```python
from build123d import *

# Parameters (mm, degrees)
BOSS_EXTRUDE1_DEPTH = 22
SKETCH4_R           = 1.25
CUT_EXTRUDE1_DEPTH  = 3
BOSS_EXTRUDE2_DEPTH = 27
BOSS_EXTRUDE3_START = 27
BOSS_EXTRUDE3_DEPTH = 11.1
BOSS_EXTRUDE5_DEPTH = 23.5
SKETCH8_R           = 1.25
CUT_EXTRUDE2_DEPTH  = 3
SKETCH9_W           = 14
SKETCH9_H           = 10.1
CUT_EXTRUDE3_DEPTH  = 3


with BuildPart() as part:
    # Sketch3 → Boss-Extrude1 (new body)
    with BuildSketch(Plane.XY):
        with BuildLine():
            Line((-15, 3), (-4.369210455, 3))
            ThreePointArc((-4.369210455, 3), (0, 5.3), (4.369210455, 3))
            Line((4.369210455, 3), (15, 3))
            Line((15, 3), (15, 6))
            Line((15, 6), (5.734980384, 6))
            ThreePointArc((5.734980384, 6), (0, 8.3), (-5.734980384, 6))
            Line((-5.734980384, 6), (-15, 6))
            Line((-15, 6), (-15, 3))
        make_face()
    extrude(amount=BOSS_EXTRUDE1_DEPTH)

    # Sketch4 → Cut-Extrude1 (cut)
    with BuildSketch(Plane(origin=(0, 6, 0), x_dir=(1, 0, 0), z_dir=(0, 1, 0))):
        with Locations(Location((11.75, -18.75, 0), (0, 0, 180))):
            Circle(SKETCH4_R)
        with Locations(Location((11.75, -3.25, 0), (0, 0, 180))):
            Circle(SKETCH4_R)
        with Locations(Location((-11.75, -3.25, 0), (0, 0, 180))):
            Circle(SKETCH4_R)
        with Locations(Location((-11.75, -18.75, 0), (0, 0, 180))):
            Circle(SKETCH4_R)
    extrude(amount=-CUT_EXTRUDE1_DEPTH, mode=Mode.SUBTRACT)

    # Sketch5 → Boss-Extrude2 (add)
    with BuildSketch(Plane.XY.offset(22)):
        with BuildLine():
            Line((6, 4), (6, 3))
            Line((6, 3), (15, 3))
            Line((15, 3), (15, 6))
            Line((15, 6), (5.734980384, 6))
            ThreePointArc((5.734980384, 6), (0, 8.3), (-5.734980384, 6))
            Line((-5.734980384, 6), (-15, 6))
            Line((-15, 6), (-15, 3))
            Line((-15, 3), (-6, 3))
            Line((-6, 3), (-6, 4))
            ThreePointArc((-6, 4), (-5.707106781, 4.707106781), (-5, 5))
            Line((-5, 5), (-1.757839583, 5))
            ThreePointArc((-1.757839583, 5), (0, 5.3), (1.757839583, 5))
            Line((1.757839583, 5), (5, 5))
            ThreePointArc((5, 5), (5.707106781, 4.707106781), (6, 4))
        make_face()
        with BuildLine():
            ThreePointArc((-4.369210455, 3), (-3.222605397, 4.207708932), (-1.757839583, 5))
            Line((-1.757839583, 5), (-5, 5))
            ThreePointArc((-5, 5), (-5.707106781, 4.707106781), (-6, 4))
            Line((-6, 4), (-6, 3))
            Line((-6, 3), (-4.369210455, 3))
        make_face()
        with BuildLine():
            Line((4.369210455, 3), (6, 3))
            Line((6, 3), (6, 4))
            ThreePointArc((6, 4), (5.707106781, 4.707106781), (5, 5))
            Line((5, 5), (1.757839583, 5))
            ThreePointArc((1.757839583, 5), (3.222605397, 4.207708932), (4.369210455, 3))
        make_face()
    extrude(amount=BOSS_EXTRUDE2_DEPTH)

    # Sketch5<3> → Boss-Extrude3 (add)
    with BuildSketch(Plane.XY.offset(22).offset(BOSS_EXTRUDE3_START)):
        with BuildLine():
            Line((6, 4), (6, 3))
            Line((6, 3), (15, 3))
            Line((15, 3), (15, 6))
            Line((15, 6), (5.734980384, 6))
            ThreePointArc((5.734980384, 6), (0, 8.3), (-5.734980384, 6))
            Line((-5.734980384, 6), (-15, 6))
            Line((-15, 6), (-15, 3))
            Line((-15, 3), (-6, 3))
            Line((-6, 3), (-6, 4))
            ThreePointArc((-6, 4), (-5.707106781, 4.707106781), (-5, 5))
            Line((-5, 5), (-1.757839583, 5))
            ThreePointArc((-1.757839583, 5), (0, 5.3), (1.757839583, 5))
            Line((1.757839583, 5), (5, 5))
            ThreePointArc((5, 5), (5.707106781, 4.707106781), (6, 4))
        make_face()
    extrude(amount=BOSS_EXTRUDE3_DEPTH)

    # Sketch7 → Boss-Extrude5 (add)
    with BuildSketch(Plane.XY.offset(60.1)):
        with BuildLine():
            Line((-15, 6), (-15, 3))
            Line((-15, 3), (-6, 3))
            Line((-6, 3), (-6, 4))
            ThreePointArc((-6, 4), (-5.707106781, 4.707106781), (-5, 5))
            Line((-5, 5), (-1.757839583, 5))
            ThreePointArc((-1.757839583, 5), (0, 5.3), (1.757839583, 5))
            Line((1.757839583, 5), (5, 5))
            ThreePointArc((5, 5), (5.707106781, 4.707106781), (6, 4))
            Line((6, 4), (6, 3))
            Line((6, 3), (15, 3))
            Line((15, 3), (15, 6))
            Line((15, 6), (5.734980384, 6))
            ThreePointArc((5.734980384, 6), (0, 8.3), (-5.734980384, 6))
            Line((-5.734980384, 6), (-15, 6))
        make_face()
        with BuildLine():
            ThreePointArc((-5.196152423, 3), (-4.372281323, 4.108911782), (-3.31662479, 5))
            Line((-3.31662479, 5), (-5, 5))
            ThreePointArc((-5, 5), (-5.707106781, 4.707106781), (-6, 4))
            Line((-6, 4), (-6, 3))
            Line((-6, 3), (-5.196152423, 3))
        make_face()
        with BuildLine():
            Line((5, 5), (3.31662479, 5))
            ThreePointArc((3.31662479, 5), (4.372281323, 4.108911782), (5.196152423, 3))
            Line((5.196152423, 3), (6, 3))
            Line((6, 3), (6, 4))
            ThreePointArc((6, 4), (5.707106781, 4.707106781), (5, 5))
        make_face()
        with BuildLine():
            Line((-1.757839583, 5), (1.757839583, 5))
            ThreePointArc((1.757839583, 5), (0, 5.3), (-1.757839583, 5))
        make_face()
    extrude(amount=BOSS_EXTRUDE5_DEPTH)

    # Sketch8 → Cut-Extrude2 (cut)
    with BuildSketch(Plane(origin=(0, 6, 0), x_dir=(1, 0, 0), z_dir=(0, 1, 0))):
        with Locations(Location((-11.75, -80.35, 0), (0, 0, 180))):
            Circle(SKETCH8_R)
        with Locations(Location((-11.75, -50.25, 0), (0, 0, 180))):
            Circle(SKETCH8_R)
        with Locations(Location((11.75, -50.25, 0), (0, 0, 180))):
            Circle(SKETCH8_R)
        with Locations(Location((11.75, -80.35, 0), (0, 0, 180))):
            Circle(SKETCH8_R)
    extrude(amount=-CUT_EXTRUDE2_DEPTH, mode=Mode.SUBTRACT)

    # Sketch9 → Cut-Extrude3 (cut)
    with BuildSketch(Plane.XZ.offset(-3)):
        with Locations((0, 56.05)):
            Rectangle(SKETCH9_W, SKETCH9_H)
    extrude(amount=-CUT_EXTRUDE3_DEPTH, mode=Mode.SUBTRACT)


solid = part.part
```
For this review, take the finished solid that the model builds, in its own axes (mm). A direction names the side the tool comes from. Round coordinates to 2 decimals unless told otherwise and drop trailing zeros. Write each loop counter-clockwise with the first axis right and the second up, starting at its lowest first coordinate (ties: lowest second). Pieces come first, ordered by that corner, then holes. Notation, with made-up numbers: (6.5, 35.5) -> (26.5, 35.5) arc R18 cw to (26.5, 54.5) -> close; hole circle Ø7 at (82, -11). An arc over 180 degrees is marked (long way). One line per question, with ' | ' between items. Start each with the question number.
(1) Add section D-D, the plane z = 80.35. Write out the cut boundary in (x, y).
(2) For line 1 along Z through (x, y) = (11.75, 5.4); line 2 along X through (y, z) = (5.4, 80.35); line 3 along Y through (x, z) = (-13.25, 76), list the stretches that pass through material, from the lowest coordinate up. Write a range as from..to.
(3) Tool access review of faces 1 (the face through (-0.1, 5.3, 25.1)), 2 (the face through (7, 4, 56)), 3 (the face through (10, 6, 41)): name each direction out of +Z, -Z, +X, -X, +Y, -Y from which nothing blocks a thin tool from reaching the whole face with its end or side.
(4) Mouldability with a two-part tool opening along X and no side actions: class faces 4 (the face through (0.1, 8.3, 41.2)), 5 (the face through (-4.39, 4.09, 72.19)), 6 (the face through (-15, 5, 41)), 7 (the face through (-3, 5, 50)) as released by +X, released by -X, zero draft, split by the parting line, or undercut.
(5) Add section B-B, the plane z = 3.25. Write out the cut boundary in (x, y).
(6) Add section A-A, the plane x = -11.75. Write out the cut boundary in (y, z).
(7) Add section C-C, the plane z = 32.5. Write out the cut boundary in (x, y), plus the area to 3 significant figures.
(8) Insertion check: P1, Ø1.5, axis at x = -11.75, z = 80.35, coming from the +Y side; P2, Ø1.5, axis at y = 7.5, z = 24, coming from the +X side; P3, Ø1, axis at x = 4, z = 50.5, coming from the -Y side; P4, Ø1.5, axis at x = -8.5, z = 72.5, coming from the +Y side. Each pin has a flat end and moves straight along its axis. Give the tip position at first contact, or say it passes through.
Answer list:
1) outline: (-15, 3) -> (-13, 3) -> (-13, 6) -> (-15, 6) -> close; (-10.5, 3) -> (-5.2, 3) arc R6 cw to (-3.32, 5) -> (3.32, 5) arc R6 cw to (5.2, 3) -> (10.5, 3) -> (10.5, 6) -> (5.73, 6) arc R8.3 ccw to (-5.73, 6) -> (-10.5, 6) -> close; (13, 3) -> (15, 3) -> (15, 6) -> (13, 6) -> close
2) line 1: 0..2, 4.5..17.5, 20..49, 51.5..79.1, 81.6..83.6 | line 2: -15..-13, -10.5..10.5, 13..15 | line 3: 3..6
3) face 1: -Z, -Y | face 2: +Y, -Y | face 3: +Z, -Z, +X, +Y
4) face 4: split by the parting line | face 5: undercut | face 6: released by -X | face 7: undercut
5) outline: (-15, 3) -> (-13, 3) -> (-13, 6) -> (-15, 6) -> close; (-10.5, 3) -> (-4.37, 3) arc R5.3 cw to (4.37, 3) -> (10.5, 3) -> (10.5, 6) -> (5.73, 6) arc R8.3 ccw to (-5.73, 6) -> (-10.5, 6) -> close; (13, 3) -> (15, 3) -> (15, 6) -> (13, 6) -> close
6) outline: (3, 0) -> (6, 0) -> (6, 2) -> (3, 2) -> close; (3, 4.5) -> (6, 4.5) -> (6, 17.5) -> (3, 17.5) -> close; (3, 20) -> (6, 20) -> (6, 49) -> (3, 49) -> close; (3, 51.5) -> (6, 51.5) -> (6, 79.1) -> (3, 79.1) -> close; (3, 81.6) -> (6, 81.6) -> (6, 83.6) -> (3, 83.6) -> close
7) outline: (-15, 3) -> (-4.37, 3) arc R5.3 cw to (4.37, 3) -> (15, 3) -> (15, 6) -> (5.73, 6) arc R8.3 ccw to (-5.73, 6) -> (-15, 6) -> close | area: 94.0 mm²
8) P1: through | P2: x = 4.83 | P3: y = 5 | P4: y = 6
